Autodesk Inventor part; units mm, degrees
ref_plane "YZ Plane" through (0, 0, 0) normal (1, 0, 0) x (0, 1, 0)
ref_plane "XZ Plane" through (0, 0, 0) normal (0, 1, 0) x (-1, 0, 0)
ref_plane "XY Plane" through (0, 0, 0) normal (0, 0, 1) x (1, 0, 0)
sketch "Boceto1" plane through (0, 0, 0) normal (0, 1, 0) x (-1, 0, 0)
  line L0 (200, 85) -> (-200, 85)
  line L1 (-200, 85) -> (-200, -85)
  line L2 (-200, -85) -> (200, -85)
  line L3 (200, -85) -> (200, 85)
  line L4 (200, 85) -> (-200, -85) construction
  line L5 (-200, 85) -> (200, -85) construction
  point P0 (0, 0)
  dimension "d0" = 400
  dimension "d1" = 170
extrude "Extrusión1" add sketch "Boceto1" along normal blind 10
sketch "Boceto2" plane through (0, 10, 0) normal (0, 1, 0) x (1, 0, 0)
  line L0 (0, 0) -> (-100, 0)
  line L1 (0, 0) -> (100, 0) construction
  circle A0 centre (-100, 0) radius 60
  line L2 (0, 0) -> (0, 85)
  line L3 (200, 85) -> (-200, 85)
  circle A1 centre (100, 0) radius 60
  dimension "d5" = 100
  dimension "d6" = 180
  dimension "d7" = 120
extrude "Extrusión2" cut sketch "Boceto2" against normal up to surface (10 mm away)
sketch "Boceto3" plane through (0, 10, 0) normal (0, 1, 0) x (1, 0, 0)
  line L0 (165, 50) -> (235, 50)
  line L1 (235, 50) -> (235, -50)
  line L2 (235, -50) -> (165, -50)
  line L3 (165, -50) -> (165, 50)
  line L4 (200, -85) -> (200, 85)
  line L5 (165, 50) -> (235, -50) construction
  line L6 (235, 50) -> (165, -50) construction
  line L7 (200, 50) -> (200, -50)
  line L8 (0, -85) -> (0, 85)
  line L9 (200, 85) -> (-200, 85)
  line L10 (-165, 50) -> (-235, 50)
  line L11 (-235, 50) -> (-235, -50)
  line L12 (-235, -50) -> (-165, -50)
  line L13 (-200, -85) -> (-200, 85)
  point P0 (0, 0)
  point P1 (200, 0)
  point P2 (-200, -50)
  point P3 (-200, 50)
  dimension "d10" = 70
  dimension "d11" = 100
extrude "Extrusión3" add sketch "Boceto3" against normal up to surface (10 mm away) contours L13 L12 L11 L10 | L0 L1 L2 L4
sketch "Boceto4" plane through (0, 10, 0) normal (0, 1, 0) x (1, 0, 0)
  line L0 (0, 0) -> (0, 85)
  line L1 (200, 85) -> (-200, 85)
  line L2 (-235, 50) -> (-235, -50)
  line L3 (-235, 0) -> (-217.5, 0)
  line L4 (-235, 0) -> (-217.5, 0) construction
  line L5 (-222.5, -25) -> (-212.5, -25)
  line L6 (-212.5, -25) -> (-212.5, 25)
  line L7 (-212.5, 25) -> (-222.5, 25)
  line L8 (-222.5, 25) -> (-222.5, -25)
  line L9 (-222.5, -25) -> (-212.5, 25) construction
  line L10 (-212.5, -25) -> (-222.5, 25) construction
  line L11 (222.5, -25) -> (212.5, -25)
  line L12 (212.5, -25) -> (212.5, 25)
  line L13 (212.5, 25) -> (222.5, 25)
  line L14 (222.5, 25) -> (222.5, -25)
  dimension "d14" = 17.5
  dimension "d15" = 0
  dimension "d16" = 10
  dimension "d17" = 50
extrude "Extrusión4" cut sketch "Boceto4" against normal up to surface (10 mm away)
equation "\"d0\" = largo_c"
equation "\"d1\" = ancho_c"
equation "\"d2\" = grueso"
equation "\"d5\" = d_plato"
equation "\"d7\" = diametro_c"
equation "\"d10\" = largo_p"
equation "\"d11\" = ancho_p"
equation "\"d14\" = 0.25 * largo_p"
equation "\"d16\" = ancho_a"
equation "\"d17\" = alto_a"
equation "\"ancho_c\" = 170"
equation "\"largo_c\" = 400"
equation "\"grueso\" = 10"
equation "\"diametro_c\" = 120"
equation "\"d_plato\" = 100"
equation "\"ancho_p\" = 100"
equation "\"largo_p\" = 70"
equation "\"ancho_a\" = 10"
equation "\"alto_a\" = 50"
properties part number "Parte C" material "Madera (abedul)"
Read the model definition and answer for the solid it produces. Units are mm, in the model's axes. A direction names the side the tool comes from. Coordinates: 2 decimals unless noted, no trailing zeros. Order: outer loops, then holes, each group sorted by start corner. A loop starts at its lowest first (then second) coordinate and runs counter-clockwise, first axis right, second up. Notation, with made-up numbers: (17, 75) -> (75, 75) arc R11 ccw to (75, 86) -> close; hole circle Ø8 at (20, 64). An arc over 180 degrees is marked (long way). Answer as a JSON object with one key per item and string values.
1) Consider line 1 along X through (y, z) = (6, 0); line 2 along Z through (x, y) = (100, 6.25); line 3 along X through (y, z) = (6.75, -15). Determine where each line is inside the solid, lowest interval first. Write a range as from..to.
Model answer:
{"line 1": "x = -235..-222.5, -212.5..-160, -40..40, 160..212.5, 222.5..235", "line 2": "z = -85..-60, 60..85", "line 3": "x = -235..-222.5, -212.5..-158.09, -41.91..41.91, 158.09..212.5, 222.5..235"}
2) A cutting plane is placed at C-C, the plane y = 2.5. Determine the outline of the cut face in (x, z), plus the area to 3 significant figures.
Model answer:
{"outline": "(-235, -50) -> (-200, -50) -> (-200, -85) -> (200, -85) -> (200, -50) -> (235, -50) -> (235, 50) -> (200, 50) -> (200, 85) -> (-200, 85) -> (-200, 50) -> (-235, 50) -> close; hole (-222.5, -25) -> (-212.5, -25) -> (-212.5, 25) -> (-222.5, 25) -> close; hole circle Ø120 at (-100, 0); hole circle Ø120 at (100, 0); hole (212.5, -25) -> (222.5, -25) -> (222.5, 25) -> (212.5, 25) -> close", "area": "51,400 mm²"}
3) A cutting plane is placed at B-B, the plane z = 0. Determine the outline of the cut face in (x, y).
Model answer:
{"outline": "(-235, 0) -> (-222.5, 0) -> (-222.5, 10) -> (-235, 10) -> close; (-212.5, 0) -> (-160, 0) -> (-160, 10) -> (-212.5, 10) -> close; (-40, 0) -> (40, 0) -> (40, 10) -> (-40, 10) -> close; (160, 0) -> (212.5, 0) -> (212.5, 10) -> (160, 10) -> close; (222.5, 0) -> (235, 0) -> (235, 10) -> (222.5, 10) -> close"}
4) A cutting plane is placed at A-A, the plane x = 100. Determine the outline of the cut face in (y, z).
Model answer:
{"outline": "(0, -85) -> (10, -85) -> (10, -60) -> (0, -60) -> close; (0, 60) -> (10, 60) -> (10, 85) -> (0, 85) -> close"}
5) A cutting plane is placed at D-D, the plane z = -44.5. Determine the outline of the cut face in (x, y).
Model answer:
{"outline": "(-235, 0) -> (-140.25, 0) -> (-140.25, 10) -> (-235, 10) -> close; (-59.75, 0) -> (59.75, 0) -> (59.75, 10) -> (-59.75, 10) -> close; (140.25, 0) -> (235, 0) -> (235, 10) -> (140.25, 10) -> close"}
6) Each of these flat-tipped pins is pushed along its axis until it touches: pin 1 (3 mm diameter, centred on x = -217, y = 3.5, fed in from +Z); pin 2 (5 mm diameter, centred on x = -217, y = 7.5, fed in from -Z); pin 3 (3 mm diameter, centred on y = 3.5, z = 65, fed in from +X). Where does it stop, or does it pass through?
Model answer:
{"pin 1": "stops at z = 50", "pin 2": "stops at z = -50", "pin 3": "stops at x = 200"}
7) A tool of negligible diameter and unlimited length cuts with its end or side. For faces 5 (the face through (218, 5, 50)), 6 (the face through (200, 5, -67)), 7 (the face through (-200, 5, -68)), from which of +Z, -Z, +X, -X, +Y, -Y can it reach the whole face along a straight path? Write none if from no direction.
Model answer:
{"face 5": "+Z, +X, +Y, -Y", "face 6": "-Z, +X, +Y, -Y", "face 7": "-Z, -X, +Y, -Y"}
8) The mould has two halves that part along Z. Classify faces 1 (the face through (-218, 5, 50)), 2 (the face through (3, 0, 1)), 3 (the face through (218, 5, 25)), 4 (the face through (222.5, 5, 0)): released by +Z, released by -Z, zero draft, split by the parting line, or undercut.
Model answer:
{"face 1": "released by +Z", "face 2": "zero draft", "face 3": "undercut", "face 4": "undercut"}
